The listing builds one solid part. Answer for the finished solid, in the listing's coordinates (mm). A direction names the side the tool comes from. Give positions to 0.01 mm unless a question says otherwise; leave off trailing zeros. Order: outer loops, then holes, each group sorted by start corner. A loop starts at its lowest first (then second) coordinate and runs counter-clockwise, first axis right, second up. Notation, with made-up numbers: (58.25, 25) - (80.25, 25) arc R14 cw to (80.25, 31) - close; hole circle Ø3 at (63.25, 32.5). An arc over 180 degrees is marked (long way). Answer in a Markdown table with one row per item.
from build123d import *

# Parameters (mm, degrees)
F0_R     = 6.1
F1_DEPTH = 15
F4_R     = 1.089334
F5_DEPTH = 5


with BuildPart() as f1:
    # F0 (on Top) → F1 (new body)
    with BuildSketch(Plane.XY):
        Circle(F0_R)
    extrude(amount=F1_DEPTH)

    # F2 (on Front) → F3 (revolve, cut)
    with BuildSketch(Plane.XZ):
        Polygon((0, 4.542232), (0, 0), (1.185742, 0), align=None)
        Polygon((0, 4.542232), (1.185742, 0), (2.746811, 0), align=None)
    revolve(axis=Axis((0, 0, 2.271116), (0, 0, -1)), mode=Mode.SUBTRACT)

    # F4 (on face) → F5 (cut)
    with BuildSketch(Plane(origin=(0, 0, 0), x_dir=(1, 0, 0), z_dir=(0, 0, -1))):
        Circle(F4_R)
    extrude(amount=-F5_DEPTH, mode=Mode.SUBTRACT)


solid = f1.part
Item 1: Determine the mould class of faces 3 (the face through (3, -1, 0)), 4 (the face through (-0.236, 1.063, 3.855)), 5 (the face through (-6.094, 0.268, 7.395)) for opening direction Y: pulls with the +Y half, pulls with the -Y half, needs draft (parallel to the pull), parting line crosses it, or undercut.
Answer block:
| item | result |
|---|---|
| face 3 | needs draft |
| face 4 | undercut |
| face 5 | parting line crosses it |
Item 2: Find section D-D on z = 10.25. Write down the section's boundary in (x, y), then the cut area to 3 significant figures.
Answer block:
| item | result |
|---|---|
| outline | circle Ø12.2 at (0, 0) |
| area | 117 mm² |
Item 3: Consider line 1 (Y direction, x = 0, z = 3.7); line 2 (Y direction, x = 0, z = 2.5) (3 decimals); line 3 (X direction, y = -1.5, z = 7). Determine where each line is inside the solid, lowest interval first.
Answer block:
| item | result |
|---|---|
| line 1 | -6.1 to -1.09, 1.09 to 6.1 |
| line 2 | -6.1 to -1.235, 1.235 to 6.1 |
| line 3 | -5.91 to 5.91 |
Item 4: Find section A-A on x = 0. Write down the section's boundary in (y, z).
Answer block:
| item | result |
|---|---|
| outline | (-6.1, 0) - (-2.75, 0) - (-1.09, 2.74) - (-1.09, 5) - (1.09, 5) - (1.09, 2.74) - (2.75, 0) - (6.1, 0) - (6.1, 15) - (-6.1, 15) - close |
Item 5: Find section C-C on z = 4.75. Write down the section's boundary in (x, y), then the cut area to 3 significant figures.
Answer block:
| item | result |
|---|---|
| outline | circle Ø12.2 at (0, 0); hole circle Ø2.18 at (0, 0) |
| area | 113 mm² |
Item 6: Which of the six approach directions +Z, -Z, +X, -X, +Y, -Y give full straight-line access (tool end or side, diameter ignored) to faces 1 (the face through (0, 0, 15)), 2 (the face through (0, 0, 5))?
Answer block:
| item | result |
|---|---|
| face 1 | +Z, +X, -X, +Y, -Y |
| face 2 | -Z |
Item 7: Each of these flat-tipped pins is pushed along its axis until it touches: P1, Ø5, axis at y = -4.5, z = 11, coming from the +X side; P2, Ø1.5, axis at x = 3.5, z = 3, coming from the +Y side; P3, Ø3, axis at y = -2, z = 2, coming from the +X side. Where does it stop, or does it pass through?
Answer block:
| item | result |
|---|---|
| P1 | x = 5.76 |
| P2 | y = 5.44 |
| P3 | x = 6.08 |
